Could you check a few things on this model? Use its own coordinates, in mm. A direction names the side the tool comes from. Give positions to 0.01 mm unless a question says otherwise; leave off trailing zeros. Loops run counter-clockwise (first coordinate to the right, second up) from the corner with the lowest first, then second, coordinate; pieces in that order, holes last. Notation, with made-up numbers: M 11,40.5 L 32,40.5 A11 ccw 32,54.5 Z; hole C -0.75,-19.5 d3. An arc over 180 degrees is marked long. Write each question's results on one line, items separated by ' | '. Start each with the question number.
from build123d import *

# Parameters (mm, degrees)
F0_R     = 11.1125
F3_DEPTH = 9.525
F1_R     = 2.921
F4_DEPTH = 12.7
F2_R     = 2.921
F5_DEPTH = 12.7
F6_R     = 0.254


with BuildPart() as f3:
    # F0 (on Front) → F3 (new body, symmetric)
    with BuildSketch(Plane.XZ):
        Circle(F0_R)
    extrude(amount=F3_DEPTH, both=True)

    # F1 (on Front) → F4 (join, symmetric)
    with BuildSketch(Plane.XZ):
        Circle(F1_R)
    extrude(amount=F4_DEPTH, both=True)

    # F2 (on Right) → F5 (cut, symmetric)
    with BuildSketch(Plane.YZ):
        Circle(F2_R)
    extrude(amount=F5_DEPTH, both=True, mode=Mode.SUBTRACT)

    # F6
    f6_edges = [f3.edges().sort_by_distance(p)[0] for p in [
        (-2.921, -12.7, 0),
        (-11.1125, -9.525, 0),
        (-11.1125, 9.525, 0),
        (-2.921, 12.7, 0),
    ]]
    fillet(f6_edges, radius=F6_R)


solid = f3.part
1) Thinking about a two-plate mould opening in Y: for faces 1 (the face through (0.154, -0.633, -2.852)), 2 (the face through (2.3, 9.525, -2.3)), 3 (the face through (0, -12.7, 0)), which applies, pulls with the +Y half, pulls with the -Y half, needs draft (parallel to the pull), parting line crosses it, or undercut?
2) If we section it at C-C on y = 3.5: Write out the boundary of the cut face in (x, z) (1 decimal), plus the area to 3 significant figures.
3) I'm going to push flat-ended pins straight in: P1, Ø4, axis at x = -2.5, y = -7.5, coming from the +Z side; P2, Ø5, axis at x = -8, y = -3, coming from the +Z side; P3, Ø2, axis at x = 1.5, z = 8, coming from the +Y side (3 decimals). Where does each tip first touch, or does it pass through?
4) Please list where these lines run through material, in increasing order: line 1 (Y direction, x = 3.5, z = 0) (3 decimals); line 2 (Y direction, x = -2, z = 0); line 3 (Z direction, x = -0.25, y = 0). Write a range as from..to.
5) If we section it at D-D on y = 0: Write out the boundary of the cut face in (x, z) (1 decimal), plus the area to 3 significant figures.
6) Which directions (+Z, -Z, +X, -X, +Y, -Y) give clear straight access to the entire face, cutting with the end or side of a thin tool? Please do faces 4 (the face through (-0.633, 10.965, -2.852)), 5 (the face through (10.6, -0.13, 3.34)), 6 (the face through (2.3, -9.525, -2.3)).
Calculated:
1) face 1: undercut | face 2: pulls with the +Y half | face 3: pulls with the -Y half
2) outline: C 0,0 d22.2 | area: 388 mm2
3) P1: stops at z = 11.1 | P2: stops at z = 9.66 | P3: stops at y = 9.525
4) line 1: y = -9.525..-2.921, 2.921..9.525 | line 2: y = -12.7..-2.92, 2.92..12.7 | line 3: z = -11.11..-2.92, 2.92..11.11
5) outline: M -10.7,-2.9 A11.1 ccw 10.7,-2.9 Z; M -10.7,2.9 L 10.7,2.9 A11.1 ccw Z | area: 260 mm2
6) face 4: +Y | face 5: +Y, -Y | face 6: -Y
